Geometry check sheet. Reference: drawing and pictorial views, mm from the part's lowest x, y, z. A direction names the side the tool comes from. Give positions to 0.01 mm unless a question says otherwise; leave off trailing zeros. Write each loop counter-clockwise with the first axis right and the second up, starting at its lowest first coordinate (ties: lowest second). Pieces come first, ordered by that corner, then holes.
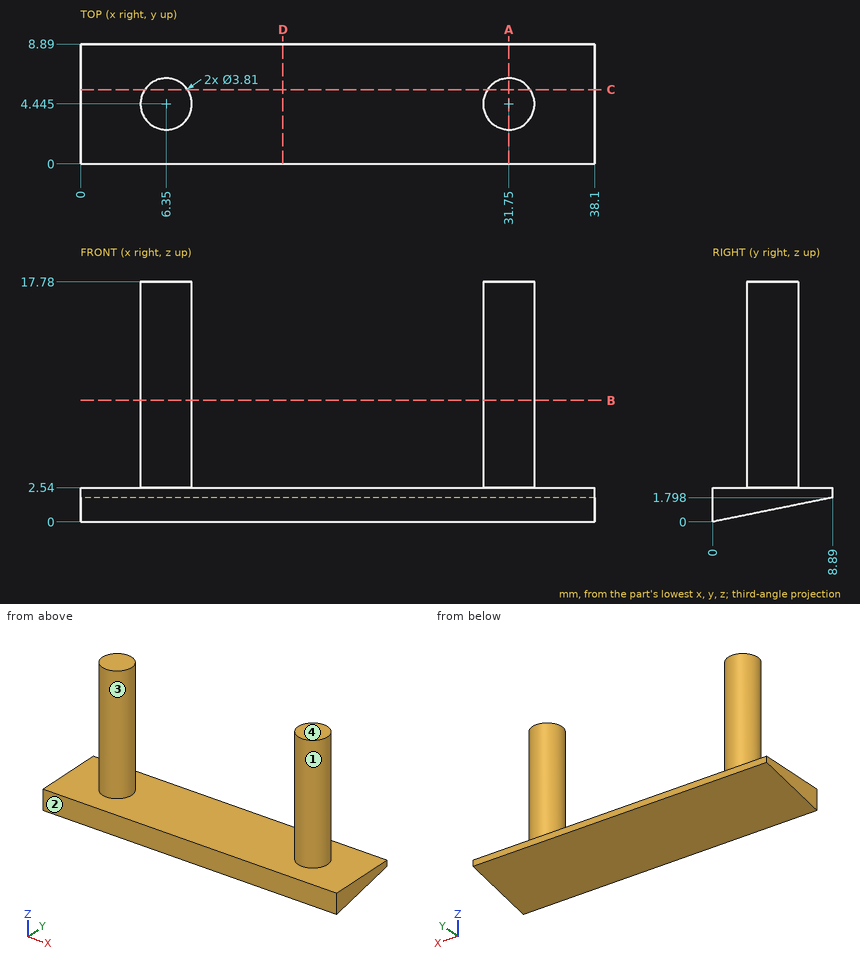
Item 1: Sectioned sample at A-A on x = 31.75. Record the cut outline in (y, z).
Answer key:
outline: (0, 0) - (8.89, 1.8) - (8.89, 2.54) - (6.35, 2.54) - (6.35, 17.78) - (2.54, 17.78) - (2.54, 2.54) - (0, 2.54) - close
Item 2: Sectioned sample at B-B on z = 9. Record the cut outline in (x, y) (3 decimals).
Answer key:
outline: circle Ø3.81 at (6.35, 4.445); circle Ø3.81 at (31.75, 4.445)
Item 3: Depth check by flat-ended pin: pin 1 (1 mm diameter, centred on x = 26.5, y = 4.5, fed in from +Z); pin 2 (3 mm diameter, centred on y = 7.5, z = 12, fed in from -X); pin 3 (8 mm diameter, centred on x = 13, z = 13, fed in from -Y). Enter the tip coordinate at first touch or a pass-through.
Answer key:
pin 1: stops at z = 2.54
pin 2: stops at x = 5.25
pin 3: passes through
Item 4: Scan lines: line 1 along X through (y, z) = (4, 16.25); line 2 along Z through (x, y) = (34.5, 3.25); line 3 along Y through (x, z) = (30, 6.75). Record each from-to range of solid material in increasing order.
Answer key:
line 1: x = 4.5 to 8.2, 29.9 to 33.6
line 2: z = 0.66 to 2.54
line 3: y = 3.69 to 5.2
Item 5: Set-up check for the marked faces 3 and 4: record each of +Z, -Z, +X, -X, +Y, -Y from which the full face is reachable in a straight line by a thin tool's end or side.
Answer key:
face 3: +Z
face 4: +Z, +X, -X, +Y, -Y
Item 6: Release check for a two-part mould opening along X. For the marked faces 1 and 2 record: released by +X, released by -X, zero draft, split by the parting line, or undercut.
Answer key:
face 1: undercut
face 2: zero draft
Item 7: Sectioned sample at C-C on y = 5.5. Record the cut outline in (x, z).
Answer key:
outline: (0, 1.11) - (38.1, 1.11) - (38.1, 2.54) - (33.34, 2.54) - (33.34, 17.78) - (30.16, 17.78) - (30.16, 2.54) - (7.94, 2.54) - (7.94, 17.78) - (4.76, 17.78) - (4.76, 2.54) - (0, 2.54) - close
Item 8: Sectioned sample at D-D on x = 15. Record the cut outline in (y, z), then the cut area to 3 significant figures.
Answer key:
outline: (0, 0) - (8.89, 1.8) - (8.89, 2.54) - (0, 2.54) - close
area: 14.6 mm2
